Build history of the part. All positions in model axes, mm. Face numbers are marked on the shaded views. A direction names the side the tool comes from. Coordinates: 2 decimals unless noted, no trailing zeros. Loops run counter-clockwise (first coordinate to the right, second up) from the corner with the lowest first, then second, coordinate; pieces in that order, holes last.
(1) Slice it at C-C (y = -22). Give the cut face in (x, z).
(2) Slice it at D-D (z = 10). Give the cut face in (x, y), and give its area (3 significant figures).
(3) Slice it at A-A (x = 0). Give the cut face in (y, z), and give its area (3 significant figures).
(4) Two-plate mould, pull along Z, no slides. Class the marked faces 1, 2, 3 and 4: pulls with the +Z half, pulls with the -Z half, needs draft (parallel to the pull), parting line crosses it, or undercut.
(5) Tool access for the marked faces 5 and 6: list every direction of +Z, -Z, +X, -X, +Y, -Y with a clear straight run to the whole face (end or side of a thin tool).
(6) Slice it at B-B (z = -2). Give the cut face in (x, y).
(7) Wall check: L1, parallel to Z at x = 0, y = -27; L2, parallel to Y at x = 5, z = 18.5; L3, parallel to X at y = -2, z = 2.5. Give the ranges that are in metal, low to high.
(8) Flat gauge pins, fed straight in: P1, Ø2, axis at y = -35.5, z = 3, coming from the +X side; P2, Ø3, axis at x = 10.5, y = -7, coming from the -Z side; P3, Ø1.5, axis at x = 7.5, z = 4.5, coming from the +Y side; P4, Ø12, axis at y = -7, z = -14, coming from the -X side. Where does each tip first touch, or does it go through?
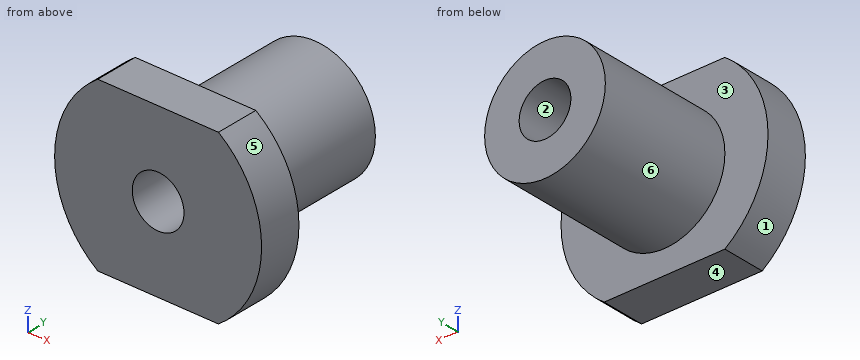
from build123d import *

# Parameters (mm, degrees)
F0_R     = 14
F1_DEPTH = 42
F2_R     = 6
F3_DEPTH = 42
F4_R     = 24
F4_R_2   = 14
F5_DEPTH = 10
F7_DEPTH = 10


with BuildPart() as f1:
    # F0 (on Front) → F1 (new body)
    with BuildSketch(Plane.XZ):
        Circle(F0_R)
    extrude(amount=F1_DEPTH)

    # F2 (on face) → F3 (cut, through all)
    with BuildSketch(Plane.XZ.offset(42)):
        Circle(F2_R)
    extrude(amount=-F3_DEPTH, mode=Mode.SUBTRACT)

    # F4 (on face) → F5 (join)
    with BuildSketch(Plane.XZ.offset(42)):
        Circle(F4_R)
        Circle(F4_R_2, mode=Mode.SUBTRACT)
    extrude(amount=-F5_DEPTH)

    # F6 (on face) → F7 (cut, through all)
    with BuildSketch(Plane.XZ.offset(42)):
        with BuildLine():
            ThreePointArc((13.9910685796, 19.5), (0, 24), (-13.9910685796, 19.5))
            Line((-13.9910685796, 19.5), (13.9910685796, 19.5))
        make_face()
        with BuildLine():
            Line((13.9910685796, -19.5), (-13.9910685796, -19.5))
            ThreePointArc((-13.9910685796, -19.5), (0, -24), (13.9910685796, -19.5))
        make_face()
    extrude(amount=-F7_DEPTH, mode=Mode.SUBTRACT)


solid = f1.part
Response values:
1. outline: circle Ø28 at (0, 0); hole circle Ø12 at (0, 0)
2. outline: (-21.82, -42) - (21.82, -42) - (21.82, -32) - (9.8, -32) - (9.8, 0) - (-9.8, 0) - (-9.8, -32) - (-21.82, -32) - close
2. area: 1,060 mm2
3. outline: (-42, -19.5) - (-32, -19.5) - (-32, -14) - (0, -14) - (0, -6) - (-42, -6) - close; (-42, 6) - (0, 6) - (0, 14) - (-32, 14) - (-32, 19.5) - (-42, 19.5) - close
3. area: 782 mm2
4. face 1: parting line crosses it
4. face 2: undercut
4. face 3: needs draft
4. face 4: pulls with the -Z half
5. face 5: +X, +Y, -Y
5. face 6: +Y
6. outline: (-23.92, -42) - (-5.66, -42) - (-5.66, 0) - (-13.86, 0) - (-13.86, -32) - (-23.92, -32) - close; (5.66, -42) - (23.92, -42) - (23.92, -32) - (13.86, -32) - (13.86, 0) - (5.66, 0) - close
7. L1: z = -14 to -6, 6 to 14
7. L2: y = -42 to -32
7. L3: x = -13.77 to -5.45, 5.45 to 13.77
8. P1: stops at x = 23.92
8. P2: stops at z = -10.72
8. P3: stops at y = 0
8. P4: stops at x = -11.49
